from build123d import *

# Parameters (mm, degrees)
F0_R      = 4
F1_DEPTH  = 5.5
F2_R      = 5
F3_DEPTH  = 3
F4_R      = 10
F5_DEPTH  = 2.5
F6_SIZE   = 1
F7_SIZE   = 0.5
F8_R      = 0.2
F9_SIZE   = 0.5
F12_START = 1.5
F11_R     = 1.45
F12_DEPTH = 10.1


with BuildPart() as f1:
    # F0 (on Top) → F1 (new body)
    with BuildSketch(Plane.XY):
        Circle(F0_R)
    extrude(amount=F1_DEPTH)

    # F2 (on Top) → F3 (join)
    with BuildSketch(Plane.XY):
        Circle(F2_R)
    extrude(amount=F3_DEPTH)

    # F4 (on Top) → F5 (join)
    with BuildSketch(Plane.XY):
        Circle(F4_R)
    extrude(amount=F5_DEPTH)

    # F6
    f6_edges = [f1.edges().sort_by_distance(p)[0] for p in [
        (-10, 0, 0),
    ]]
    chamfer(f6_edges, length=F6_SIZE)

    # F7
    f7_edges = [f1.edges().sort_by_distance(p)[0] for p in [
        (-10, 0, 2.5),
    ]]
    chamfer(f7_edges, length=F7_SIZE)

    # F8
    f8_edges = [f1.edges().sort_by_distance(p)[0] for p in [
        (-10, 0, 1),
        (-10, 0, 2),
    ]]
    fillet(f8_edges, radius=F8_R)

    # F9
    f9_edges = [f1.edges().sort_by_distance(p)[0] for p in [
        (-4, 0, 5.5),
    ]]
    chamfer(f9_edges, length=F9_SIZE)


with BuildPart() as f10_1:
    # F10: copy of F1
    add(f1.part.moved(Location((-25, 0, 0))))


with BuildPart() as f1_1:
    add(f1.part)

    # F11 (on Top) → F12 (cut)
    with BuildSketch(Plane.XY.offset(F12_START)):
        Circle(F11_R)
    extrude(amount=F12_DEPTH, mode=Mode.SUBTRACT)


with BuildPart() as f14_1:
    # F14: copy of F1
    add(f1_1.part.moved(Location((-23.4, 0, 0))))


solid = f1_1.part
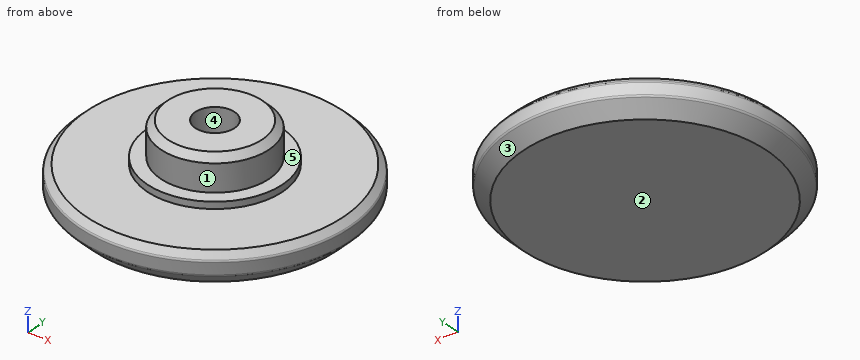
Can you work these out from the model? Positions are in its coordinate system, mm. Face numbers are marked on the shaded views. A direction names the side the tool comes from. Coordinates: 2 decimals unless noted, no trailing zeros. Order: outer loops, then holes, each group sorted by start corner. A loop starts at its lowest first (then second) coordinate and runs counter-clockwise, first axis right, second up. Notation, with made-up numbers: (14.25, 53.25) - (53.25, 53.25) arc R34 cw to (53.25, 88.25) - close; hole circle Ø3 at (57.25, 39). An arc over 180 degrees is marked (long way). Answer as a JSON object with one key per item and string values. Group by question number.
Q1. I need wall thicknesses on line 1 (Y direction, x = 0, z = 2.75); line 2 (Y direction, x = 0, z = 3.25). Which ranges of each line are inside material? Lowest first, please. Write a range as from..to.
Q2. On a 3-axis mill with a long thin cutter (end or side, diameter ignored), from which of +Z, -Z, +X, -X, +Y, -Y can I reach the whole of each face in a straight line? I mean the marked faces 1 and 2. Say none if no direction works.
Q3. Imagine slicing it at A-A (z = 4). Please give me the cut outline in (x, y).
Q4. We'd pull the mould along Y, two halves only. Please class the marked faces 3, 4 and 5: +Y half, -Y half, draft (parallel to the pull), parting line (faces both ways), or undercut.
Q5. Will this pin go through, and if not, where does the flat tip stop? P1, Ø3, axis at x = -5.5, z = 1.5, coming from the -Y side.
Determined:
{
 "1": {"line 1": "y = -5..-1.45, 1.45..5", "line 2": "y = -4..-1.45, 1.45..4"},
 "2": {"face 1": "+Z", "face 2": "-Z, +X, -X, +Y, -Y"},
 "3": {"outline": "circle Ø8 at (0, 0); hole circle Ø2.9 at (0, 0)"},
 "4": {"face 3": "parting line", "face 4": "undercut", "face 5": "draft"},
 "5": {"P1": "stops at y = -9.17"}
}
